Could you check a few things on this model? Use its own coordinates, in mm. A direction names the side the tool comes from. Coordinates: 2 decimals unless noted, no trailing zeros. Order: outer loops, then holes, each group sorted by start corner. A loop starts at its lowest first (then second) coordinate and runs counter-clockwise, first axis right, second up. Notation, with made-up numbers: (5, -0.5) - (37, -0.5) arc R31 cw to (37, 24.5) - close; hole circle Ø10 at (36, 27). An arc over 180 degrees is marked (long way). Answer as a JSON object with one key per item and string values. Group by question number.
(1) Imagine slicing it at B-B, the plane z = -12.7. Write out the boundary of the cut face in (x, y) (3 decimals).
(2) Which directions (+Z, -Z, +X, -X, +Y, -Y) give clear straight access to the entire face, cutting with the end or side of a thin tool? Please do faces 4 (the flat face through (3.175, 13, -17)), 5 (the cylindrical face through (1.61, 6.04, -9.37)).
(3) Imagine slicing it at A-A, the plane x = 9.7. Write out the boundary of the cut face in (y, z) (3 decimals).
(4) We'd pull the mould along Z, two halves only. Please class faces 1 (the cylindrical face through (1.6, 11.8, -5.5)), 2 (the flat face through (24, 13, -25.4)), 3 (the cylindrical face through (5.5, 11.8, -1.6)): pulls with the +Z half, pulls with the -Z half, needs draft (parallel to the pull), parting line crosses it, or undercut.
(5) Imagine slicing it at D-D, the plane y = 19. Give the number of separate pieces and of enclosed holes in the cut face, and give its area (3 significant figures).
(6) Please list where these lines run through material, in increasing order: probe 1 along Y at (x, z) = (15.7, -1.25); probe 2 along X at (y, z) = (14.75, -14.5) (3 decimals); probe 3 along Y at (x, z) = (2.3, -12.7).
(7) Imagine slicing it at C-C, the plane z = -9.7. Write out the boundary of the cut face in (x, y) (3 decimals), and give its area (3 significant figures).
(8) Will this pin go through, and if not, where does the flat tip stop? P1, Ø5, axis at y = 10, z = -4.5, coming from the -X side.
from build123d import *

# Parameters (mm, degrees)
BOSS_EXTRUDE1_DEPTH = 25.4
SKETCH3_R           = 1.5
CUT_EXTRUDE1_DEPTH  = 44.994090512
SKETCH4_R           = 1.5
CUT_EXTRUDE2_DEPTH  = 44.994090512


with BuildPart() as part:
    # Sketch2 → Boss-Extrude1 (new body)
    with BuildSketch(Plane(origin=(0, 0, 0), x_dir=(1, 0, 0), z_dir=(0, 1, 0))):
        Polygon((22.225, 3.175), (12.7, 3.175), (3.175, 3.175), (3.175, 25.4), (0, 25.4), (0, 0), (25.4, 0), (25.4, 25.4), (22.225, 25.4), align=None)
    extrude(amount=BOSS_EXTRUDE1_DEPTH)

    # Sketch3 → Cut-Extrude1 (cut, through all)
    with BuildSketch(Plane.XY):
        with Locations((12.7, 12.7)):
            Circle(SKETCH3_R)
        with Locations((6.7, 12.7)):
            Circle(SKETCH3_R)
        with Locations((9.7, 17.896152423)):
            Circle(SKETCH3_R)
        with Locations((15.7, 17.896152423)):
            Circle(SKETCH3_R)
        with Locations((18.7, 12.7)):
            Circle(SKETCH3_R)
        with Locations((15.7, 7.503847577)):
            Circle(SKETCH3_R)
        with Locations((9.7, 7.503847577)):
            Circle(SKETCH3_R)
    extrude(amount=-CUT_EXTRUDE1_DEPTH, mode=Mode.SUBTRACT)

    # Sketch4 → Cut-Extrude2 (cut, through all)
    with BuildSketch(Plane(origin=(25.4, 0, 0), x_dir=(0, 0, -1), z_dir=(1, 0, 0))):
        with Locations((12.7, 12.7)):
            Circle(SKETCH4_R)
        with Locations((6.7, 12.7)):
            Circle(SKETCH4_R)
        with Locations((9.7, 17.896152423)):
            Circle(SKETCH4_R)
        with Locations((15.7, 17.896152423)):
            Circle(SKETCH4_R)
        with Locations((18.7, 12.7)):
            Circle(SKETCH4_R)
        with Locations((15.7, 7.503847577)):
            Circle(SKETCH4_R)
        with Locations((9.7, 7.503847577)):
            Circle(SKETCH4_R)
    extrude(amount=-CUT_EXTRUDE2_DEPTH, mode=Mode.SUBTRACT)


solid = part.part
Result set:
{
 "1": {"outline": "(0, 0) - (3.175, 0) - (3.175, 11.2) - (0, 11.2) - close; (0, 14.2) - (3.175, 14.2) - (3.175, 25.4) - (0, 25.4) - close; (22.225, 0) - (25.4, 0) - (25.4, 11.2) - (22.225, 11.2) - close; (22.225, 14.2) - (25.4, 14.2) - (25.4, 25.4) - (22.225, 25.4) - close"},
 "2": {"face 4": "-Z, +Y, -Y", "face 5": "+X, -X"},
 "3": {"outline": "(0, -3.175) - (6.004, -3.175) - (6.004, 0) - (0, 0) - close; (9.004, -3.175) - (16.396, -3.175) - (16.396, 0) - (9.004, 0) - close; (19.396, -3.175) - (25.4, -3.175) - (25.4, 0) - (19.396, 0) - close"},
 "4": {"face 1": "undercut", "face 2": "pulls with the -Z half", "face 3": "needs draft"},
 "5": {"separate pieces": "7", "enclosed holes": "0", "area": "183 mm^2"},
 "6": {"probe 1": "y = 0 to 6, 9 to 16.4, 19.4 to 25.4", "probe 2": "x = 0 to 3.175, 22.225 to 25.4", "probe 3": "y = 0 to 11.2, 14.2 to 25.4"},
 "7": {"outline": "(0, 0) - (3.175, 0) - (3.175, 6.004) - (0, 6.004) - close; (0, 9.004) - (3.175, 9.004) - (3.175, 16.396) - (0, 16.396) - close; (0, 19.396) - (3.175, 19.396) - (3.175, 25.4) - (0, 25.4) - close; (22.225, 0) - (25.4, 0) - (25.4, 6.004) - (22.225, 6.004) - close; (22.225, 9.004) - (25.4, 9.004) - (25.4, 16.396) - (22.225, 16.396) - close; (22.225, 19.396) - (25.4, 19.396) - (25.4, 25.4) - (22.225, 25.4) - close", "area": "123 mm^2"},
 "8": {"P1": "stops at x = 0"}
}
